from build123d import *

# Parameters (mm, degrees)
F0_W      = 50
F0_H      = 20
F1_DEPTH  = 3
F3_DEPTH  = 10
F4_DEPTH  = 10
F5_W      = 2.5
F5_H      = 20
F5_W_2    = 5
F6_DEPTH  = 6
F7_W      = 14
F7_H      = 3
F8_DEPTH  = 25
F9_W      = 14
F9_H      = 3
F10_DEPTH = 25
F12_DEPTH = 10
F13_DEPTH = 10
F14_R     = 0.99999
F15_R     = 1
F16_W     = 2.5
F16_H     = 20
F17_DEPTH = 25
F18_W     = 2.5
F18_H     = 20
F19_DEPTH = 25
F20_R     = 0.99999


# Not quite as in the source:
# - a fillet or chamfer is up to 0.001 mm smaller than in the source, because OpenCascade refuses the exact size


with BuildPart() as f1:
    # F0 (on Top) → F1 (new body)
    with BuildSketch(Plane.XY):
        Rectangle(F0_W, F0_H)
    extrude(amount=F1_DEPTH)

    # F2 (on Front) → F3 (join)
    with BuildSketch(Plane.XZ):
        Polygon((0, 0), (-22, 0), (-22, -2.1), align=None)
        Polygon((22, 0), (0, 0), (22, -2.1), align=None)
    extrude(amount=F3_DEPTH)

    # F4 (add): faces of the model
    f4_faces = [f1.faces().sort_by_distance(p)[0] for p in [
        (14.6666666667, 0, -0.7),
        (-14.6666666667, 0, -0.7),
    ]]
    extrude(f4_faces, amount=F4_DEPTH)

    # F5 (on face) → F6 (join)
    with BuildSketch(Plane.XY.offset(3)):
        with Locations((-23.75, 0)):
            Rectangle(F5_W, F5_H)
        with Locations((-20, 0)):
            Rectangle(F5_W_2, F5_H)
        with Locations((23.75, 0)):
            Rectangle(F5_W, F5_H)
        with Locations((20, 0)):
            Rectangle(F5_W_2, F5_H)
    extrude(amount=F6_DEPTH)

    # F7 (on face) → F8 (cut)
    with BuildSketch(Plane.YZ.offset(-17.5)):
        with Locations((0, 4.5)):
            Rectangle(F7_W, F7_H)
    extrude(amount=-F8_DEPTH, mode=Mode.SUBTRACT)

    # F9 (on face) → F10 (cut)
    with BuildSketch(Plane(origin=(17.5, 0, 0), x_dir=(0, -1, 0), z_dir=(-1, 0, 0))):
        with Locations((0, 4.5)):
            Rectangle(F9_W, F9_H)
    extrude(amount=-F10_DEPTH, mode=Mode.SUBTRACT)

    # F11 (on Front) → F12 (join)
    with BuildSketch(Plane.XZ):
        with BuildLine():
            Line((-10, 10), (-10, 3))
            Line((-10, 3), (10, 3))
            Line((10, 3), (10, 10))
            ThreePointArc((10, 10), (0, 6.5968126209), (-10, 10))
        make_face()
    extrude(amount=F12_DEPTH)

    # F13 (add): a face of the model
    f13_faces = [f1.faces().sort_by_distance(p)[0] for p in [
        (0, 0, 5.4458216504),
    ]]
    extrude(f13_faces, amount=F13_DEPTH)

    # F14 (radius 1 in the source; OpenCascade refuses exactly that, so slightly less here)
    f14_edges = [f1.edges().sort_by_distance(p)[0] for p in [
        (-17.5, 0, 9),
        (-25, 0, 0),
        (-22, 0, 0),
        (-22, 0, -2.1),
        (25, 0, 0),
        (22, 0, 0),
        (22, 0, -2.1),
        (17.5, 0, 9),
        (17.5, 0, 6),
        (25, 0, 6),
        (25, -7, 4.5),
        (17.5, -7, 4.5),
        (25, 7, 4.5),
        (17.5, 7, 4.5),
        (25, 0, 3),
        (-25, 0, 6),
        (-17.5, -7, 4.5),
        (-25, -7, 4.5),
        (-25, 0, 3),
        (-17.5, 0, 6),
        (-17.5, 7, 4.5),
    ]]
    fillet(f14_edges, radius=F14_R)

    # F15
    f15_edges = [f1.edges().sort_by_distance(p)[0] for p in [
        (-10, 0, 10),
        (10, 0, 10),
    ]]
    fillet(f15_edges, radius=F15_R)

    # F16 (on face) → F17 (cut)
    with BuildSketch(Plane.XY.offset(9)):
        with Locations((-23.75, 0)):
            Rectangle(F16_W, F16_H)
    extrude(amount=-F17_DEPTH, mode=Mode.SUBTRACT)

    # F18 (on face) → F19 (cut)
    with BuildSketch(Plane.XY.offset(9)):
        with Locations((23.75, 0)):
            Rectangle(F18_W, F18_H)
    extrude(amount=-F19_DEPTH, mode=Mode.SUBTRACT)

    # F20 (radius 1 in the source; OpenCascade refuses exactly that, so slightly less here)
    f20_edges = [f1.edges().sort_by_distance(p)[0] for p in [
        (-22.5, 0, -0.13397),
        (22.5, 0, -0.13397),
        (22.5, 0, 9),
        (20.499995, -10, 9),
        (20.499995, 10, 9),
        (-20.499995, 10, 9),
        (-22.5, 0, 9),
        (-20.499995, -10, 9),
    ]]
    fillet(f20_edges, radius=F20_R)


solid = f1.part
The listing builds one solid part. Answer for the finished solid, in the listing's coordinates (mm). A direction names the side the tool comes from. Coordinates: 2 decimals unless noted, no trailing zeros. Write each loop counter-clockwise with the first axis right and the second up, starting at its lowest first coordinate (ties: lowest second). Pieces come first, ordered by that corner, then holes. Notation, with made-up numbers: (28, 22) - (70, 22) arc R20 ccw to (70, 36) - close; hole circle Ø3 at (-6.75, -14.75). An arc over 180 degrees is marked (long way). Put each result on its own line as item: value.
1. The part is cut by section D-D on x = 19. Give the vertices of the cut face in (y, z), plus the area to 3 significant figures.
Answer sheet:
outline: (-10, -1.81) - (10, -1.81) - (10, 8) arc R1 ccw to (9, 9) - (-9, 9) arc R1 ccw to (-10, 8) - close; hole (-7, 3) - (7, 3) - (7, 6) - (-7, 6) - close
area: 174 mm^2
2. Determine the mould class of faces 1 (the face through (0, 10, 2)), 2 (the face through (-21.66, 0.14, -1.75)), 3 (the face through (17.801, -7.285, 4.584)) for opening direction Y: pulls with the +Y half, pulls with the -Y half, needs draft (parallel to the pull), parting line crosses it, or undercut.
Answer sheet:
face 1: pulls with the +Y half
face 2: needs draft
face 3: undercut
3. The part is cut by section C-C on z = 7.5. Give the vertices of the cut face in (x, y).
Answer sheet:
outline: (-22.5, -10) - (-18.5, -10) arc R1 ccw to (-17.5, -9) - (-17.5, 9) arc R1 ccw to (-18.5, 10) - (-22.5, 10) - close; (-10, -10) - (-5.37, -10) - (-5.37, 10) - (-10, 10) - close; (5.37, -10) - (10, -10) - (10, 10) - (5.37, 10) - close; (17.5, -9) arc R1 ccw to (18.5, -10) - (22.5, -10) - (22.5, 10) - (18.5, 10) arc R1 ccw to (17.5, 9) - close
4. The part is cut by section A-A on z = 4. Give the vertices of the cut face in (x, y), plus the area to 3 significant figures.
Answer sheet:
outline: (-22.5, -10) - (-18.5, -10) arc R1 ccw to (-17.5, -9) - (-17.5, -8) arc R1 ccw to (-18.5, -7) - (-22.5, -7) - close; (-22.5, 7) - (-18.5, 7) arc R1 ccw to (-17.5, 8) - (-17.5, 9) arc R1 ccw to (-18.5, 10) - (-22.5, 10) - close; (-10, -10) - (10, -10) - (10, 10) - (-10, 10) - close; (17.5, -9) arc R1 ccw to (18.5, -10) - (22.5, -10) - (22.5, -7) - (18.5, -7) arc R1 ccw to (17.5, -8) - close; (17.5, 8) arc R1 ccw to (18.5, 7) - (22.5, 7) - (22.5, 10) - (18.5, 10) arc R1 ccw to (17.5, 9) - close
area: 458 mm^2
5. The part is cut by section B-B on y = -6.25. State how many separate pieces and enclosed holes the cut face has, plus the area to 3 significant figures.
Answer sheet:
separate pieces: 3
enclosed holes: 0
area: 302 mm^2
6. Flat-ended cylindrical pins translate along their axes: pin 1 Ø1.5 at (x, z) = (12.5, 4) entering from -Y; pin 2 Ø2.5 at (y, z) = (4.5, 4.5) entering from -X; pin 3 Ø1.5 at (x, y) = (5, 0.5) entering from -Z; pin 4 Ø2.5 at (x, y) = (-20.5, -4) entering from +Z. Find the tip coordinate at first contact, or state that the pin passes through.
Answer sheet:
pin 1: passes through
pin 2: stops at x = -10
pin 3: stops at z = -0.55
pin 4: stops at z = 9
7. Find the intervals of material crossed by line 1 along Z through (x, y) = (0, 6); line 2 along Y through (x, z) = (19, 3.25); line 3 along X through (y, z) = (4.5, 8.75), in increasing order. Write a range as from..to.
Answer sheet:
line 1: z = 0..6.6
line 2: y = -10..-7, 7..10
line 3: x = -22.16..-17.84, -9.77..-8.12, 8.12..9.77, 17.84..22.16
8. A tool of negligible diameter and unlimited length cuts with its end or side. For faces 4 (the face through (-16, 0, 3)), 5 (the face through (20, -7, 4)), 6 (the face through (-10.6, -0.14, -1.01)), from which of +Z, -Z, +X, -X, +Y, -Y can it reach the whole face along a straight path? Write none if from no direction.
Answer sheet:
face 4: none
face 5: +X
face 6: -Z, +Y, -Y
